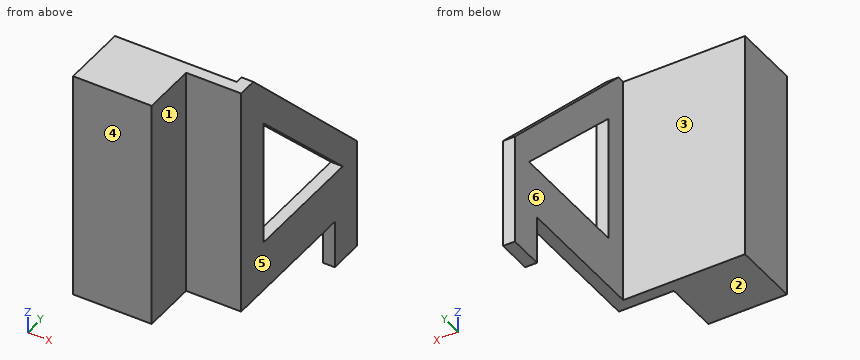
```python
from build123d import *

# Parameters (mm, degrees)
SKETCH_2_W          = 17
SKETCH_2_H          = 35
EXTRUDE_1_DEPTH     = 1.5
SKETCH_3_W          = 10
SKETCH_3_H          = 35
EXTRUDE_2_DEPTH     = 7
SKETCH_4_W          = 1.5
SKETCH_4_H          = 35.577657925
EXTRUDE_3_DEPTH     = 22
CUT_EXTRUDE_1_REACH = 47.902
CUT_EXTRUDE_2_REACH = 47.902
SKETCH_11_W         = 17
SKETCH_11_H         = 6.846873931
CUT_EXTRUDE_7_DEPTH = 26


with BuildPart() as part:
    # 草图2 → 凸台-拉伸1 (new body)
    with BuildSketch(Plane(origin=(0, 0, 0), x_dir=(1, 0, 0), z_dir=(0, 1, 0))):
        with Locations((8.5, 17.5)):
            Rectangle(SKETCH_2_W, SKETCH_2_H)
    extrude(amount=EXTRUDE_1_DEPTH)

    # 草图3 → 凸台-拉伸2 (add)
    with BuildSketch(Plane.XZ):
        with Locations((5, -17.5)):
            Rectangle(SKETCH_3_W, SKETCH_3_H)
    extrude(amount=EXTRUDE_2_DEPTH)

    # 草图4 → 凸台-拉伸3 (add)
    with BuildSketch(Plane(origin=(0, 1.5, 0), x_dir=(1, 0, 0), z_dir=(0, 1, 0))):
        with Locations((16.25, 17.788828963)):
            Rectangle(SKETCH_4_W, SKETCH_4_H)
    extrude(amount=EXTRUDE_3_DEPTH)

    # 草图7 → 切除-拉伸1 (cut, up to next)
    with BuildSketch(Plane(origin=(17, 0, 0), x_dir=(0, 0, -1), z_dir=(1, 0, 0)), mode=Mode.PRIVATE) as cut_extrude_1_sk1:
        Polygon((0, 23.5), (0, 2.460497923), (21.413333868, 23.5), align=None)
    cut_extrude_1_tool1 = extrude(cut_extrude_1_sk1.sketch, amount=-CUT_EXTRUDE_1_REACH, mode=Mode.PRIVATE) & part.part
    add(cut_extrude_1_tool1.solids().sort_by_distance((17, 16.486833, -7.137778))[0], mode=Mode.SUBTRACT)

    # 草图8 → 切除-拉伸2 (cut, up to next)
    with BuildSketch(Plane(origin=(17, 0, 0), x_dir=(0, 0, -1), z_dir=(1, 0, 0)), mode=Mode.PRIVATE) as cut_extrude_2_sk1:
        Polygon((22.994680785, 20.618265403), (6.90545418, 4.529038798), (22.994680785, 4.529038798), align=None)
    cut_extrude_2_tool1 = extrude(cut_extrude_2_sk1.sketch, amount=-CUT_EXTRUDE_2_REACH, mode=Mode.PRIVATE) & part.part
    add(cut_extrude_2_tool1.solids().sort_by_distance((17, 9.892114, -17.631605))[0], mode=Mode.SUBTRACT)

    # 草图11 → 切除-拉伸7 (cut)
    with BuildSketch(Plane.XZ.offset(7)):
        with Locations((8.5, -32.86825369)):
            Rectangle(SKETCH_11_W, SKETCH_11_H)
    extrude(amount=-CUT_EXTRUDE_7_DEPTH, mode=Mode.SUBTRACT)


solid = part.part
```
Design review of the part built by this model. Coordinates are the model's own, in mm. Face numbers are marked on the shaded views. A direction names the side the tool comes from. Give positions to 0.01 mm unless a question says otherwise; leave off trailing zeros. Order: outer loops, then holes, each group sorted by start corner. A loop starts at its lowest first (then second) coordinate and runs counter-clockwise, first axis right, second up. Notation, with made-up numbers: (66, 37) -> (117, 37) arc R25 cw to (117, 63) -> close; hole circle Ø5 at (48.5, -1). An arc over 180 degrees is marked (long way). Write each question's results on one line, items separated by ' | '. Start each with the question number.
Q1. Add section B-B on y = 10. Give the boundary of the cut face in (x, z), and give its area (3 significant figures).
Q2. Mouldability with a two-part tool opening along X and no side actions: class the marked faces 4, 5 and 6 as +X half, -X half, draft (parallel to the pull), parting line (faces both ways), or undercut.
Q3. Add section D-D on x = 10.5. Give the boundary of the cut face in (y, z), and give its area (3 significant figures).
Q4. Wall thickness on L1, parallel to Y at x = 8.5, z = -10; L2, parallel to X at y = 4, z = -21.5; L3, parallel to Y at x = 13.75, z = -16: over which ranges is each line inside the solid? List them lowest first. Write a range as from..to.
Q5. Add section C-C on z = -20. Give the boundary of the cut face in (x, y), and give its area (3 significant figures).
Q6. Machinability: for the marked faces 1, 2 and 3, which of the approach directions +Z, -Z, +X, -X, +Y, -Y give a long, thin tool a straight path to every point of the face, cutting with its end or side? Answer none if there is none.
Q7. Add section A-A on z = -28.5. Give the boundary of the cut face in (x, y), and give its area (4 significant figures).
Q8. For pin 1 (5 mm diameter, centred on x = 14.5, z = -22.5, fed in from -Y); pin 2 (1.6 mm diameter, centred on x = 16, z = -16.5, fed in from +Y); pin 3 (5 mm diameter, centred on x = 5, z = -14, fed in from +Y), all flat-tipped, find the tip position at first contact; note any pin that passes through.
Found:
1) outline: (15.5, -29.44) -> (17, -29.44) -> (17, -22.99) -> (15.5, -22.99) -> close; (15.5, -12.38) -> (17, -12.38) -> (17, -7.67) -> (15.5, -7.67) -> close | area: 16.7 mm2
2) face 4: draft | face 5: +X half | face 6: -X half
3) outline: (0, -29.44) -> (1.5, -29.44) -> (1.5, 0) -> (0, 0) -> close | area: 44.2 mm2
4) L1: y = -7..1.5 | L2: x = 15.5..17 | L3: y = 0..1.5
5) outline: (0, -7) -> (10, -7) -> (10, 0) -> (17, 0) -> (17, 4.53) -> (15.5, 4.53) -> (15.5, 1.5) -> (0, 1.5) -> close; (15.5, 17.62) -> (17, 17.62) -> (17, 22.11) -> (15.5, 22.11) -> close | area: 107 mm2
6) face 1: +Z, -Z, +X, -Y | face 2: -Z, +X, -X, -Y | face 3: +Z, -Z, -X, +Y
7) outline: (0, -7) -> (10, -7) -> (10, 0) -> (17, 0) -> (17, 23.5) -> (15.5, 23.5) -> (15.5, 1.5) -> (0, 1.5) -> close | area: 128.5 mm2
8) pin 1: stops at y = 0 | pin 2: stops at y = 19.46 | pin 3: stops at y = 1.5
